Work out the finished part from the listing and answer in its coordinate system (mm). A direction names the side the tool comes from. Round coordinates to 2 decimals unless told otherwise and drop trailing zeros. Order: outer loops, then holes, each group sorted by start corner. A loop starts at its lowest first (then second) coordinate and runs counter-clockwise, first axis right, second up. Notation, with made-up numbers: (-29, 56.25) - (-6, 56.25) arc R14 ccw to (-6, 61.25) - close; hole circle Ø7 at (-37.5, -8.5). An arc over 180 degrees is marked (long way). One line per question, with ' | ' between items. Start each with the question number.
from build123d import *
from build123d.topology import SkipClean

# Parameters (mm, degrees)
BOSS_EXTRUDE1_DEPTH  = 10
SKETCH6_R            = 5
BOSS_EXTRUDE4_DEPTH  = 32.5
SKETCH10_W           = 10
SKETCH10_H           = 45
CUT_EXTRUDE5_DEPTH   = 10
CUT_EXTRUDE10_START  = -10
CUT_EXTRUDE10_DEPTH  = 10
BOSS_EXTRUDE8_DEPTH  = 10
SKETCH19_R           = 1.5
CUT_EXTRUDE11_DEPTH  = 110.357366333
BOSS_EXTRUDE9_DEPTH  = 16
BOSS_EXTRUDE10_DEPTH = 10
CUT_EXTRUDE12_DEPTH  = 6
SKETCH24_W           = 5
SKETCH24_H           = 45
CUT_EXTRUDE14_DEPTH  = 10


with BuildPart() as part:
    # Sketch1 → Boss-Extrude1 (new body)
    with BuildSketch(Plane.XY):
        with BuildLine():
            Line((-10, 0), (0, 0))
            Line((0, 0), (0, 70))
            ThreePointArc((0, 70), (2.048726408, 76.039631539), (7.349256082, 79.586293943))
            ThreePointArc((7.349256082, 79.586293943), (9.526416607, 79.679930085), (11.536628421, 78.838595348))
            Line((11.536628421, 78.838595348), (37.563736921, 60.412060989))
            ThreePointArc((37.563736921, 60.412060989), (44.533661589, 61.603761507), (43.341961071, 68.573686175))
            Line((43.341961071, 68.573686175), (14.637016156, 88.896060969))
            ThreePointArc((14.637016156, 88.896060969), (13.552177116, 89.478358799), (12.35793082, 89.777895591))
            ThreePointArc((12.35793082, 89.777895591), (11.217987252, 89.884880656), (10.073780788, 89.926217211))
            ThreePointArc((10.073780788, 89.926217211), (4.526251311, 89.180986887), (-0.595162082, 86.922319935))
            ThreePointArc((-0.595162082, 86.922319935), (-4.504675426, 83.740794413), (-7.490811299, 79.680081201))
            ThreePointArc((-7.490811299, 79.680081201), (-9.362505501, 75), (-10, 70))
            Line((-10, 70), (-10, 0))
        make_face()
    extrude(amount=BOSS_EXTRUDE1_DEPTH)

    # Sketch6 → Boss-Extrude4 (add)
    with BuildSketch(Plane.XY.offset(10)):
        with Locations((-5, 70)):
            Circle(SKETCH6_R)
    extrude(amount=BOSS_EXTRUDE4_DEPTH)

    # Sketch10 → Cut-Extrude5 (cut)
    with BuildSketch(Plane(origin=(0, 0, 0), x_dir=(-1, 0, 0), z_dir=(0, 0, -1))):
        with Locations((5, 22.5)):
            Rectangle(SKETCH10_W, SKETCH10_H)
    extrude(amount=-CUT_EXTRUDE5_DEPTH, mode=Mode.SUBTRACT)

    # Sketch17 → Cut-Extrude10 (cut)
    with BuildSketch(Plane.XY.offset(10).offset(CUT_EXTRUDE10_START)):
        with BuildLine():
            Line((-10, 45), (0, 45))
            Line((0, 45), (0, 70))
            ThreePointArc((0, 70), (-5, 65), (-10, 70))
            Line((-10, 70), (-10, 45))
        make_face()
    extrude(amount=CUT_EXTRUDE10_DEPTH, mode=Mode.SUBTRACT)

    # Sketch18 → Boss-Extrude8 (add)
    with SkipClean():  # the faces are left unmerged after this step: merging them gives an invalid solid
        with BuildSketch(Plane.XY.offset(42.5)):
            with BuildLine():
                Line((0, 70), (0, -25.857864376))
                ThreePointArc((0, -25.857864376), (-5, -55), (-10, -25.857864376))
                Line((-10, -25.857864376), (-10, 70))
                ThreePointArc((-10, 70), (-5, 75), (0, 70))
            make_face()
        extrude(amount=BOSS_EXTRUDE8_DEPTH)
    add(part.part.scale(1), mode=Mode.REPLACE)  # the faces are merged on a copy

    # Sketch19 → Cut-Extrude11 (cut, through all)
    with BuildSketch(Plane(origin=(0, 0, 42.5), x_dir=(-1, 0, 0), z_dir=(0, 0, -1))):
        with Locations((5, -40)):
            Circle(SKETCH19_R)
        with Locations((10.565661313, -35.754600825)):
            Circle(SKETCH19_R)
        with Locations((0.754600825, -34.434338687)):
            Circle(SKETCH19_R)
        with Locations((-0.565661313, -44.245399175)):
            Circle(SKETCH19_R)
        with Locations((9.245399175, -45.565661313)):
            Circle(SKETCH19_R)
    extrude(amount=-CUT_EXTRUDE11_DEPTH, mode=Mode.SUBTRACT)

    # Sketch20 → Boss-Extrude9 (add)
    with BuildSketch(Plane(origin=(0, 0, 0), x_dir=(-1, 0, 0), z_dir=(0, 0, -1))):
        Polygon((-52.228493699, 70.702095376), (-47.407985115, 74.274587083), (-33.118018288, 54.992552749), (-37.938526871, 51.420061042), align=None)
    extrude(amount=BOSS_EXTRUDE9_DEPTH)

    # Sketch21 → Boss-Extrude10 (add)
    with BuildSketch(Plane.XY):
        with BuildLine():
            Line((43.237723755, 68.647483557), (43.341961071, 68.573686175))
            ThreePointArc((43.341961071, 68.573686175), (44.533661589, 61.603761507), (37.563736921, 60.412060989))
            Line((37.563736921, 60.412060989), (37.282165609, 60.611406354))
            Line((37.282165609, 60.611406354), (33.118018288, 54.992552749))
            Line((33.118018288, 54.992552749), (37.938526871, 51.420061042))
            Line((37.938526871, 51.420061042), (52.228493699, 70.702095376))
            Line((52.228493699, 70.702095376), (47.407985115, 74.274587083))
            Line((47.407985115, 74.274587083), (43.237723755, 68.647483557))
        make_face()
    extrude(amount=BOSS_EXTRUDE10_DEPTH)

    # Sketch22 → Cut-Extrude12 (cut)
    with BuildSketch(Plane(origin=(-0.109097108, 0.080852156, 0), x_dir=(0, 0, -1), z_dir=(0.8034180972667123, -0.5954152844732287, 0))):
        Polygon((12.5, 71.859534489), (12.5, 79.942438258), (5.5, 83.983890142), (-1.5, 79.942438258), (-1.5, 71.859534489), (5.5, 67.818082605), align=None)
    extrude(amount=-CUT_EXTRUDE12_DEPTH, mode=Mode.SUBTRACT)

    # Sketch24 → Cut-Extrude14 (cut)
    with BuildSketch(Plane.ZY.offset(10)):
        with Locations((45, 22.071067812)):
            Rectangle(SKETCH24_W, SKETCH24_H)
    extrude(amount=-CUT_EXTRUDE14_DEPTH, mode=Mode.SUBTRACT)


solid = part.part
1) For faces 4 (the flat face through (43, 63, 1.5)), 5 (the flat face through (-5, -0.429, 45)), 6 (the flat face through (-5, -33, 42.5)), 7 (the flat face through (-10, 21, 49)), 8 (the flat face through (46.33, 67.72, -2.05)), determine the directions among +Z, -Z, +X, -X, +Y, -Y from which every point of the face is accessible in a straight line to the end or side of a thin tool.
2) Section A-A on y = -40 is taken. Give the vertices of the cut face in (x, z).
3) Section D-D on y = 14 is taken. Give the vertices of the cut face in (x, z), and give its area (3 significant figures).
4) Flat-ended cylindrical pins translate along their axes: pin 1 (1 mm diameter, centred on x = 12, z = 6.5, fed in from -Y); pin 2 (4 mm diameter, centred on x = -5.5, z = 23.5, fed in from -Y); pin 3 (4 mm diameter, centred on x = 0.57, y = -44.25, fed in from -Z); pin 4 (2.5 mm diameter, centred on x = -9.25, y = -45.57, fed in from +Z). Find the tip coordinate at first contact, or state that the pin passes through.
5) Section B-B on z = 4.5 is taken. Give the vertices of the cut face in (x, y).
6) Straight lines are drawn through the part: line 1 (X direction, y = 70, z = 3.5); line 2 (Z direction, x = 19.5, y = 81); line 3 (Z direction, x = -2, y = 30.5). For each, find the intervals that lie inside material, in ascending order.
7) Determine the mould class of faces 1 (the cylindrical face through (-8.92, -47.03, 47.43)), 2 (the flat face through (0, 23, 49)), 3 (the flat face through (39.08, 57.93, -8.95)) for opening direction Y: released by +Y, released by -Y, zero draft, split by the parting line, or undercut.
8) Section C-C on x = -5 is taken. Give the vertices of the cut face in (y, z), and give its area (3 significant figures).
Recorded:
1) face 4: none | face 5: -Z, +X, -X | face 6: -Z, +X, -X, -Y | face 7: +Z, -Z, -X, +Y | face 8: -Y
2) outline: (-20, 42.5) - (-6.5, 42.5) - (-6.5, 52.5) - (-20, 52.5) - close; (-3.5, 42.5) - (10, 42.5) - (10, 52.5) - (-3.5, 52.5) - close
3) outline: (-10, 47.5) - (0, 47.5) - (0, 52.5) - (-10, 52.5) - close | area: 50.0 mm²
4) pin 1: stops at y = 78.16 | pin 2: stops at y = 65 | pin 3: stops at z = 42.5 | pin 4: passes through
5) outline: (-10, 70) arc R5 ccw to (0, 70) arc R9.93 cw to (7.35, 79.59) arc R5 cw to (11.54, 78.84) - (37.28, 60.61) - (33.12, 54.99) - (37.94, 51.42) - (52.23, 70.7) - (47.41, 74.27) - (43.24, 68.65) - (14.64, 88.9) arc R5 ccw to (12.36, 89.78) arc R19.93 ccw to start
6) line 1: x = -10 to 0, 24.02 to 41.33, 44.24 to 51.71 | line 2: z = 0 to 10 | line 3: z = 47.5 to 52.5
7) face 1: undercut | face 2: zero draft | face 3: released by +Y
8) outline: (-55, 42.5) - (-41.5, 42.5) - (-41.5, 52.5) - (-55, 52.5) - close; (-38.5, 42.5) - (-0.43, 42.5) - (-0.43, 47.5) - (44.57, 47.5) - (44.57, 42.5) - (65, 42.5) - (65, 0) - (83.2, 0) - (83.2, 10) - (75, 10) - (75, 52.5) - (-38.5, 52.5) - close | area: 1,550 mm²
